Model file for the job. Use its own axes, mm. A direction names the side the tool comes from. Coordinates: 2 decimals unless noted, no trailing zeros. Write each loop counter-clockwise with the first axis right and the second up, starting at its lowest first coordinate (ties: lowest second). Pieces come first, ordered by that corner, then holes. Notation, with made-up numbers: (46.25, -19.75) - (56.25, -19.75) arc R22 ccw to (56.25, -5.75) - close; hole circle Ø1 at (60.25, 45.25). An arc over 180 degrees is marked (long way). Put each result on its own line as item: value. Start each with the question number.
1. Drop flat-ended pins along their axis: P1, Ø1.5, axis at x = -3.5, z = 70, coming from the -Y side; P2, Ø6, axis at x = 2.5, y = 67, coming from the -Z side; P3, Ø5, axis at x = 5.5, y = 199, coming from the -Z side. Give the stop position or say it passes through.
2. Pull direction Y, two halves, no side cores. Call faces 4 (the face through (-1, 30, 63)), 5 (the face through (-49.217, 296.17, -9.237)), 6 (the face through (-60, 69, -40)): released by +Y, released by -Y, zero draft, split by the parting line, or undercut.
3. Which spindle directions (+Z, -Z, +X, -X, +Y, -Y) get a long thin tool onto all of the face, cutting with end or side? Do faces 1 (the face through (40, 69, -60)), 2 (the face through (-99.65, 78.43, 5.38)), 3 (the face through (-12, 34, -75)). Say none if no direction does.
4. Drill centre lines: L1, parallel to Y at x = -87, z = 0; L2, parallel to Y at x = 54.5, z = 0; L3, parallel to Z at x = -51.5, y = 95.5. Where is each one in solid material? Low to high. Write a range as from..to.
5. Saw through at D-D, the plane z = 0. Give the number of separate pieces and of enclosed holes in the cut face, plus the area to 3 significant figures.
6. Saw through at C-C, the plane x = -84.5. Write the cut outline in (y, z), plus the area to 3 significant figures.
7. Saw through at B-B, the plane z = -88.5. Write the cut outline in (x, y), plus the area to 3 significant figures.
8. Saw through at A-A, the plane y = 300. Write the cut outline in (x, z).
```python
from build123d import *

# Parameters (mm, degrees)
SKETCH1_R           = 60
BOSS_EXTRUDE1_DEPTH = 380
SKETCH2_R           = 40
CUT_EXTRUDE1_DEPTH  = 300
SKETCH3_R           = 10
CUT_EXTRUDE2_DEPTH  = 150
BOSS_EXTRUDE2_START = -30
SKETCH4_W           = 150
SKETCH4_H           = 80
SKETCH4_W_2         = 80
SKETCH4_H_2         = 150
BOSS_EXTRUDE2_DEPTH = 80
SKETCH5_R           = 32.5
SKETCH5_R_2         = 10
BOSS_EXTRUDE3_DEPTH = 50
FILLET1_R           = 5
CIRPATTERN2_COUNT   = 4
FILLET2_R           = 5


with BuildPart() as part:
    # Sketch1 → Boss-Extrude1 (new body)
    with BuildSketch(Plane(origin=(0, 0, 0), x_dir=(1, 0, 0), z_dir=(0, 1, 0))):
        with Locations(Location((0, 0, 0), (0, 0, 270))):
            Circle(SKETCH1_R)
    extrude(amount=BOSS_EXTRUDE1_DEPTH)

    # Sketch2 → Cut-Extrude1 (cut)
    with BuildSketch(Plane(origin=(0, 380, 0), x_dir=(1, 0, 0), z_dir=(0, 1, 0))):
        with Locations(Location((0, 0, 0), (0, 0, 270))):
            Circle(SKETCH2_R)
    extrude(amount=-CUT_EXTRUDE1_DEPTH, mode=Mode.SUBTRACT)

    # Sketch3 → Cut-Extrude2 (cut, symmetric)
    with BuildSketch(Plane(origin=(0, 0, 0), x_dir=(0, 0, -1), z_dir=(1, 0, 0))):
        with Locations((0, 300)):
            Circle(SKETCH3_R)
    extrude(amount=CUT_EXTRUDE2_DEPTH, both=True, mode=Mode.SUBTRACT)

    # Sketch4 → Boss-Extrude2 (add)
    with BuildSketch(Plane.XZ.offset(BOSS_EXTRUDE2_START)):
        Rectangle(SKETCH4_W, SKETCH4_H)
        Rectangle(SKETCH4_W_2, SKETCH4_H_2)
    extrude(amount=-BOSS_EXTRUDE2_DEPTH)

    # Sketch5 → Boss-Extrude3 (add)
    with BuildSketch(Plane.ZY.offset(75)):
        with Locations((0, 70)):
            Circle(SKETCH5_R)
        with Locations((0, 70)):
            Circle(SKETCH5_R_2, mode=Mode.SUBTRACT)
    boss_extrude3 = extrude(amount=BOSS_EXTRUDE3_DEPTH)

    # Fillet1
    fillet1_edges = [part.edges().sort_by_distance(p)[0] for p in [
        (-75, 70, -32.5),
    ]]
    fillet(fillet1_edges, radius=FILLET1_R)

    # CirPattern2: Boss-Extrude3 ×4 about axis
    cirpattern2_axis = Axis((0, 0, 0), (0, 1, 0))
    for i in range(1, CIRPATTERN2_COUNT):
        add(boss_extrude3.rotate(cirpattern2_axis, i * 360 / CIRPATTERN2_COUNT))

    # Fillet2
    fillet2_edges = [part.edges().sort_by_distance(p)[0] for p in [
        (-32.5, 70, 75),
        (75, 70, 32.5),
        (32.5, 70, -75),
    ]]
    fillet(fillet2_edges, radius=FILLET2_R)


solid = part.part
```
Final values:
1. P1: stops at y = 30
1. P2: stops at z = -75
1. P3: stops at z = -59.92
2. face 4: released by -Y
2. face 5: undercut
2. face 6: zero draft
3. face 1: -Z, +X, +Y, -Y
3. face 2: -X
3. face 3: -Z
4. L1: y = 37.5..60, 80..102.5
4. L2: y = 0..290, 310..380
4. L3: z = -40..40
5. separate pieces: 3
5. enclosed holes: 0
5. area: 30,100 mm²
6. outline: circle Ø65 at (70, 0); hole circle Ø20 at (70, 0)
6. area: 3,000 mm²
7. outline: circle Ø65 at (0, 70); hole circle Ø20 at (0, 70)
7. area: 3,000 mm²
8. outline: (-59.16, -10) arc R60 ccw to (59.16, -10) - (38.73, -10) arc R40 cw to (-38.73, -10) - close; (-59.16, 10) - (-38.73, 10) arc R40 cw to (38.73, 10) - (59.16, 10) arc R60 ccw to start
